from build123d import *

# Parameters (mm, degrees)
ESQUISSE1_R        = 0.5
BOSS_EXTRU_1_DEPTH = 1


with BuildPart() as part:
    # Esquisse1 → Boss.-Extru.1 (new body)
    with BuildSketch(Plane.XY):
        with BuildLine():
            Line((1.25, 7), (4, 7))
            ThreePointArc((4, 7), (4.707106781, 6.707106781), (5, 6))
            Line((5, 6), (5, -6))
            ThreePointArc((5, -6), (4.707106781, -6.707106781), (4, -7))
            Line((4, -7), (1.25, -7))
            ThreePointArc((1.25, -7), (0, -5.75), (-1.25, -7))
            Line((-1.25, -7), (-4, -7))
            ThreePointArc((-4, -7), (-4.707106781, -6.707106781), (-5, -6))
            Line((-5, -6), (-5, 6))
            ThreePointArc((-5, 6), (-4.707106781, 6.707106781), (-4, 7))
            Line((-4, 7), (-1.25, 7))
            ThreePointArc((-1.25, 7), (0, 5.75), (1.25, 7))
        make_face()
        with Locations((-2.5, -0.4)):
            Circle(ESQUISSE1_R, mode=Mode.SUBTRACT)
    extrude(amount=BOSS_EXTRU_1_DEPTH)


solid = part.part
Model file for the job. Use its own axes, mm. Coordinates: 2 decimals unless noted, no trailing zeros. Write each loop counter-clockwise with the first axis right and the second up, starting at its lowest first coordinate (ties: lowest second). Pieces come first, ordered by that corner, then holes. Notation, with made-up numbers: (-37.5, -24) -> (-32.5, -24) arc R17 cw to (-32.5, -4) -> close; hole circle Ø3 at (39.25, 75). An arc over 180 degrees is marked (long way). One line per item, written item: value. Start each with the question number.
1) Slice it at B-B on x = -2.5. Write the cut outline in (y, z).
2) Slice it at C-C on z = 0.2. Write the cut outline in (x, y), then the cut area to 3 significant figures.
3) Probe probe 1 along Y at (x, z) = (-2.5, 0.25); probe 2 along X at (y, z) = (-6, 0.65); probe 3 along Y at (x, z) = (-2.75, 0.9). List the from-to ranges inside material, lowest first.
4) Slice it at A-A on y = -0.4. Write the cut outline in (x, z), then the cut area to 3 significant figures.
5) Pull direction Y, two halves, no side cores. Call faces 1 (the face through (-2.9, -0.7, 0.5)), 2 (the face through (0, 0, 1)), 3 (the face through (0.03, -5.75, 0.49)), 4 (the face through (-4.715, 6.699, 0.493)): +Y half, -Y half, draft (parallel to the pull), parting line (faces both ways), or undercut.
6) Slice it at D-D on x = 0. Write the cut outline in (y, z), then the cut area to 3 significant figures.
Answers follow:
1. outline: (-7, 0) -> (-0.9, 0) -> (-0.9, 1) -> (-7, 1) -> close; (0.1, 0) -> (7, 0) -> (7, 1) -> (0.1, 1) -> close
2. outline: (-5, -6) arc R1 ccw to (-4, -7) -> (-1.25, -7) arc R1.25 cw to (1.25, -7) -> (4, -7) arc R1 ccw to (5, -6) -> (5, 6) arc R1 ccw to (4, 7) -> (1.25, 7) arc R1.25 cw to (-1.25, 7) -> (-4, 7) arc R1 ccw to (-5, 6) -> close; hole circle Ø1 at (-2.5, -0.4)
2. area: 133 mm2
3. probe 1: -7 to -0.9, 0.1 to 7
3. probe 2: -5 to -0.75, 0.75 to 5
3. probe 3: -7 to -0.83, 0.03 to 7
4. outline: (-5, 0) -> (-3, 0) -> (-3, 1) -> (-5, 1) -> close; (-2, 0) -> (5, 0) -> (5, 1) -> (-2, 1) -> close
4. area: 9.00 mm2
5. face 1: undercut
5. face 2: draft
5. face 3: -Y half
5. face 4: +Y half
6. outline: (-5.75, 0) -> (5.75, 0) -> (5.75, 1) -> (-5.75, 1) -> close
6. area: 11.5 mm2
